The model under review builds one solid part; all positions refer to its coordinate system, in mm. A direction names the side the tool comes from. Round coordinates to 2 decimals unless told otherwise and drop trailing zeros. Write each loop counter-clockwise with the first axis right and the second up, starting at its lowest first coordinate (ties: lowest second). Pieces come first, ordered by that corner, then holes. Notation, with made-up numbers: M -2,66.5 L 40,66.5 A33 cw 40,96.5 Z; hole C 35,84.25 d10. An arc over 180 degrees is marked long. One line per item, written item: value. Start each with the question number.
1) Take a section at C-C, the plane y = -14. Write out the cut boundary in (x, z), and give its area (3 significant figures).
2) Tool access review of faces 1 (the face through (0, 37, 3.175)), 2 (the face through (-28.43, 6.67, 3.22)), 3 (the face through (-16.85, -32.39, 3.84)): name each direction out of +Z, -Z, +X, -X, +Y, -Y from which nothing blocks a thin tool from reaching the whole face with its end or side.
3) Take a section at D-D, the plane y = 20. Write out the cut boundary in (x, z) (3 decimals), and give its area (3 significant figures).
4) Mouldability with a two-part tool opening along Y and no side actions: class faces 4 (the face through (22.37, 6.67, 3.22)), 5 (the face through (-0.835, 38.065, 1.565)), 6 (the face through (-1.845, -28.627, 3.219)), 7 (the face through (1, -1, 6.35)) as +Y half, -Y half, draft (parallel to the pull), parting line (faces both ways), or undercut.
5) Wall thickness on probe 1 along X at (y, z) = (8, 3); probe 2 along X at (y, z) = (7.62, 3) (3 decimals); probe 3 along Y at (x, z) = (-25.4, 2.75) (3 decimals): over which ranges is each line inside the solid? List them lowest first.
6) For P1, Ø0.5, axis at x = 37.5, z = 1, coming from the -Y side; P2, Ø2, axis at x = 22, z = 2.5, coming from the +Y side; P3, Ø3, axis at x = -8.5, z = 1, coming from the -Y side, all flat-tipped, find the tip position at first contact; note any pin that passes through.
7) Take a section at A-A, the plane z = 1.75. State how many separate pieces and enclosed holes the cut face has, and give its area (3 significant figures).
Autodesk Fusion 360 part; units mm, degrees
sketch "Sketch1" plane through (0, 0, 0) normal (0, 0, 1) x (1, 0, 0)
  circle A0 centre (0, 0) radius 38.0746
  dimension "d1" = 76.1492
extrude "Extrude1" add sketch "Sketch1" along normal blind 3.175
sketch "Sketch2" plane through (0, 0, 3.175) normal (0, 0, 1) x (-1, 0, 0)
  circle A0 centre (0, 0) radius 38.0746
  circle A1 centre (0, 0) radius 36.5125
  dimension "d4" = 73.025
extrude "Extrude2" add sketch "Sketch2" along normal blind 3.175 contours A1
sketch "Sketch3" plane through (0, 0, 6.35) normal (0, 0, 1) x (-1, 0, 0)
  circle A0 centre (0, 0) radius 36.5125
  circle A1 centre (25.4, -7.62) radius 3.175
  circle A2 centre (-25.4, -7.62) radius 3.175
  circle A3 centre (0, 20.6756) radius 5.08
  circle A4 centre (0, 0) radius 38.0746
  dimension "d7" = 50.8
  dimension "d8" = 25.4
  dimension "d9" = 7.62
  dimension "d10" = 6.35
  dimension "d11" = 6.35
  dimension "d12" = 10.16
  dimension "d13" = 20.6756
extrude "Extrude3" cut sketch "Sketch3" against normal blind 6.35 contours A1 | A2 | A3
sketch "Sketch4" plane through (0, 0, 6.35) normal (0, 0, 1) x (-1, 0, 0)
  circle A0 centre (-25.4, -7.62) radius 3.175
  circle A1 centre (0, 20.6756) radius 5.08
  circle A2 centre (25.4, -7.62) radius 3.175
  circle A3 centre (0, 0) radius 36.5125
  line L0 (38.0746, -0.0035) -> (36.5125, -0.0035)
  line L1 (-38.0746, 0.0019) -> (-36.5125, 0.0019)
  arc A4 (38.0746, -0.0035) -> (-38.0746, 0.0019) centre (0, 0) ccw
  arc A5 (36.5125, -0.0035) -> (-36.5125, 0.0019) centre (0, 0) ccw
  circle A6 centre (0, 20.6756) radius 8.509
  dimension "d16" = 76.1492
  dimension "d17" = 73.025
  dimension "d19" = 17.018
extrude "Extrude4" cut sketch "Sketch4" against normal through all contours A3 L0 L1 A4 A5
sketch "Sketch6" plane through (0, 0, 6.35) normal (0, 0, 1) x (1, 0, 0)
  circle A0 centre (0, -20.32) radius 8.509
  dimension "d20" = 17.018
extrude "Extrude5" cut sketch "Sketch6" against normal blind 27.94
equation "d2 = ( 0.25 / 2 ) * 1 in"
equation "d5 = ( 0.25 / 2 ) * 1 in"
Checked values:
1. outline: M -33.72,0 L -5.7,0 L -5.7,6.35 L -33.72,6.35 Z; M 5.7,0 L 33.72,0 L 33.72,6.35 L 5.7,6.35 Z
1. area: 356 mm2
2. face 1: +Z, +Y
2. face 2: +Z, -Z
2. face 3: +Z
3. outline: M -32.399,0 L 32.399,0 L 32.399,3.175 L 30.548,3.175 L 30.548,6.35 L -30.548,6.35 L -30.548,3.175 L -32.399,3.175 Z
3. area: 400 mm2
4. face 4: undercut
4. face 5: +Y half
4. face 6: undercut
4. face 7: draft
5. probe 1: x = -37.22 to -28.55, -22.25 to 22.25, 28.55 to 37.22
5. probe 2: x = -37.304 to -28.575, -22.225 to 22.225, 28.575 to 37.304
5. probe 3: y = -26.23 to 4.445, 10.795 to 28.364
6. P1: stops at y = 0
6. P2: stops at y = 31.76
6. P3: stops at y = -35.84
7. separate pieces: 1
7. enclosed holes: 3
7. area: 4,080 mm2
